```python
from build123d import *

# Parameters (mm, degrees)
F0_W     = 74
F0_H     = 25
F0_R     = 7
F0_R_2   = 9.906
F1_DEPTH = 25
F3_D     = 2.4
F3_DEPTH = 10
F3_TIP   = 0.7210327428
F4_R     = 5
F5_R     = 5.5
F5_R_2   = 4.2
F6_DEPTH = 10


with BuildPart() as f1:
    # F0 (on Top) → F1 (new body)
    with BuildSketch(Plane.XY):
        Rectangle(F0_W, F0_H)
        with Locations((-15.75, 0)):
            Circle(F0_R, mode=Mode.SUBTRACT)
        with Locations((15.75, 0)):
            Circle(F0_R_2, mode=Mode.SUBTRACT)
    extrude(amount=F1_DEPTH)

    # F3
    with Locations(Plane.XZ.offset(12.5)):
        with Locations((15.752, 12.5), (-15.752, 12.5)):
            Hole(F3_D / 2, depth=F3_DEPTH)
            with Locations((0, 0, -(F3_DEPTH + F3_TIP / 2))):  # 118° drill point
                Cone(0, F3_D / 2, F3_TIP, mode=Mode.SUBTRACT)

    # F4
    f4_edges = [f1.edges().sort_by_distance(p)[0] for p in [
        (-37, -12.5, 12.5),
        (37, -12.5, 12.5),
        (37, 12.5, 12.5),
        (-37, 12.5, 12.5),
    ]]
    fillet(f4_edges, radius=F4_R)

    # F5 (on face) → F6 (join)
    with BuildSketch(Plane(origin=(0, 12.5, 0), x_dir=(-1, 0, 0), z_dir=(0, 1, 0))):
        with Locations((-16, 12.5)):
            Circle(F5_R)
        with Locations((-16, 12.5)):
            Circle(F5_R_2, mode=Mode.SUBTRACT)
        with Locations((16, 12.5)):
            Circle(F5_R)
        with Locations((16, 12.5)):
            Circle(F5_R_2, mode=Mode.SUBTRACT)
    extrude(amount=F6_DEPTH)


solid = f1.part
```
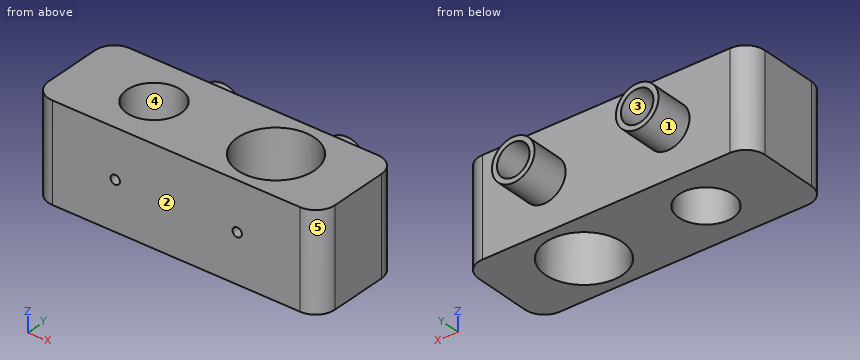
Check sheet for the modelled part. Datum: model origin and axes. Units: mm. Face numbers are marked on the shaded views. A direction names the side the tool comes from. Round coordinates to 2 decimals unless told otherwise and drop trailing zeros. Order: outer loops, then holes, each group sorted by start corner. A loop starts at its lowest first (then second) coordinate and runs counter-clockwise, first axis right, second up. Notation, with made-up numbers: (52.5, -31.75) -> (87.5, -31.75) arc R31 ccw to (87.5, -7.75) -> close; hole circle Ø6 at (57.5, -20). An arc over 180 degrees is marked (long way). Use CSV: the item, a comma, the result in double quotes.
(1) Material ranges on line 1 along X through (y, z) = (-4, 20.25); line 2 along X through (y, z) = (1.5, 13.75); line 3 along Y through (x, z) = (2.5, 20.75), recorded low to high. Write a range as from..to.
Worked out:
line 1,"-37..-21.49, -10.01..6.69, 24.81..37"
line 2,"-37..-22.59, -8.91..5.96, 25.54..37"
line 3,"-12.5..12.5"
(2) Tool access check on the marked faces 1 and 2. Record the directions out of +Z, -Z, +X, -X, +Y, -Y that give a thin tool (end or side, any length) a straight path to the whole face; none if there is none.
Worked out:
face 1,"+Y"
face 2,"+Z, -Z, +X, -X, -Y"
(3) Depth check by flat-ended pin: pin 1 (2 mm diameter, centred on x = -23, z = 5.5, fed in from +Y). Enter the tip coordinate at first touch or a pass-through.
Worked out:
pin 1,"y = 12.5"
(4) Cross-section at B-B (y = 0). Record the boundary of the cut face in (x, z), and give its area (3 significant figures).
Worked out:
outline,"(-37, 0) -> (-22.75, 0) -> (-22.75, 25) -> (-37, 25) -> close; (-8.75, 0) -> (5.84, 0) -> (5.84, 25) -> (-8.75, 25) -> close; (25.66, 0) -> (37, 0) -> (37, 25) -> (25.66, 25) -> close"
area,"1,000 mm²"
(5) Cross-section at C-C (x = -16). Record the boundary of the cut face in (y, z).
Worked out:
outline,"(-12.5, 0) -> (-7, 0) -> (-7, 11.33) -> (-12.5, 11.33) -> close; (-12.5, 13.67) -> (-7, 13.67) -> (-7, 25) -> (-12.5, 25) -> close; (7, 0) -> (12.5, 0) -> (12.5, 7) -> (22.5, 7) -> (22.5, 8.3) -> (12.5, 8.3) -> (12.5, 16.7) -> (22.5, 16.7) -> (22.5, 18) -> (12.5, 18) -> (12.5, 25) -> (7, 25) -> close"
(6) Cross-section at A-A (z = 2). Record the boundary of the cut face in (x, y).
Worked out:
outline,"(-37, -7.5) arc R5 ccw to (-32, -12.5) -> (32, -12.5) arc R5 ccw to (37, -7.5) -> (37, 7.5) arc R5 ccw to (32, 12.5) -> (-32, 12.5) arc R5 ccw to (-37, 7.5) -> close; hole circle Ø14 at (-15.75, 0); hole circle Ø19.81 at (15.75, 0)"
(7) Draft check along Y on the marked faces 3, 4 and 5. Enter one of: pulls with the +Y half, pulls with the -Y half, needs draft (parallel to the pull), parting line crosses it, or undercut.
Worked out:
face 3,"needs draft"
face 4,"undercut"
face 5,"pulls with the -Y half"
